Build history of the part. All positions in model axes, mm. Face numbers are marked on the shaded views. A direction names the side the tool comes from. Round coordinates to 2 decimals unless told otherwise and drop trailing zeros. Order: outer loops, then holes, each group sorted by start corner. A loop starts at its lowest first (then second) coordinate and runs counter-clockwise, first axis right, second up. Notation, with made-up numbers: (-14, 27.5) -> (-3, 27.5) arc R23 ccw to (-3, 39.5) -> close; hole circle Ø7 at (84, 82.5). An arc over 180 degrees is marked (long way). Use a Markdown table: item, result. Add a question column.
Item 1: Probe L1, parallel to Y at x = 23.5, z = -3; L2, parallel to Z at x = 8.75, y = -4.25; L3, parallel to X at y = -3.25, z = -17. List the from-to ranges inside material, lowest first.
Item 2: 3-axis set-ups, long thin cutter, end or side, ignore diameter. For the marked faces 1, 2, 3, 4 and 5: which of +Z, -Z, +X, -X, +Y, -Y reach the whole face in a straight line?
Item 3: Slice it at A-A, the plane x = 4.25. Give the cut face in (y, z).
Item 4: Slice it at B-B, the plane y = -3.5. Give the cut face in (x, z).
Item 5: Slice it at C-C, the plane y = -7. Give the cut face in (x, z).
Item 6: Pin check, flat tips, straight feed: pin 1 (12 mm diameter, centred on x = 18, z = -5.5, fed in from -Y); pin 2 (1 mm diameter, centred on x = 16.5, y = -4, fed in from +Z); pin 3 (1.9 mm diameter, centred on x = 12.5, y = -2.5, fed in from -Z). Stop position of each tip, or through.
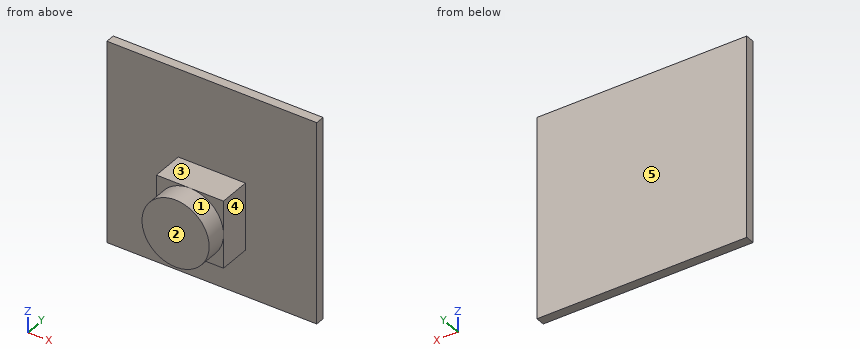
from build123d import *

# Parameters (mm, degrees)
F0_W     = 25
F0_H     = 24
F1_DEPTH = 1.1
F2_W     = 8
F2_H     = 8
F3_DEPTH = 3.8
F4_R     = 4
F5_DEPTH = 2.5


with BuildPart() as f1:
    # F0 (on Front) → F1 (new body)
    with BuildSketch(Plane.XZ):
        with Locations((12.5, -12)):
            Rectangle(F0_W, F0_H)
    extrude(amount=F1_DEPTH)

    # F2 (on face) → F3 (join)
    with BuildSketch(Plane.XZ.offset(1.1)):
        with Locations((12.5, -14.5)):
            Rectangle(F2_W, F2_H)
    extrude(amount=F3_DEPTH)

    # F4 (on face) → F5 (join)
    with BuildSketch(Plane.XZ.offset(4.9)):
        with Locations((12.5, -14.5)):
            Circle(F4_R)
    extrude(amount=F5_DEPTH)


solid = f1.part
Check sheet entries:
| question | item | result |
|---|---|---|
| 1 | L1 | -1.1 to 0 |
| 1 | L2 | -18.5 to -10.5 |
| 1 | L3 | 8.5 to 16.5 |
| 2 | face 1 | -Y |
| 2 | face 2 | +Z, -Z, +X, -X, -Y |
| 2 | face 3 | +Z, +X, -X, -Y |
| 2 | face 4 | +Z, -Z, +X, -Y |
| 2 | face 5 | +Z, -Z, +X, -X, +Y |
| 3 | outline | (-1.1, -24) -> (0, -24) -> (0, 0) -> (-1.1, 0) -> close |
| 4 | outline | (8.5, -18.5) -> (16.5, -18.5) -> (16.5, -10.5) -> (8.5, -10.5) -> close |
| 5 | outline | circle Ø8 at (12.5, -14.5) |
| 6 | pin 1 | y = -4.9 |
| 6 | pin 2 | z = -10.5 |
| 6 | pin 3 | z = -18.5 |
